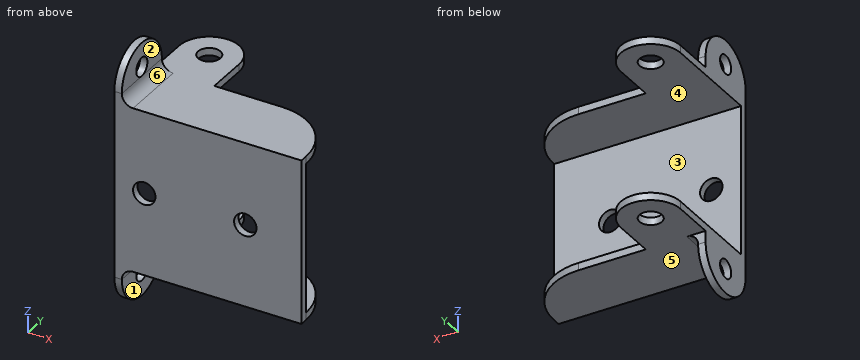
```python
from build123d import *

# Parameters (mm, degrees)
CROQUIS1_W              = 25
CROQUIS1_H              = 22
SALIENTE_EXTRUIR1_DEPTH = 1
CROQUIS2_W              = 8
CROQUIS2_H              = 1
SALIENTE_EXTRUIR2_DEPTH = 17.6
CROQUIS2_3_W            = 17
CROQUIS2_3_H            = 1
SALIENTE_EXTRUIR3_DEPTH = 8
REDONDEO2_RADIUS        = 4
REDONDEO2_LENGTH        = 1
REDONDEO3_R             = 8
REDONDEO4_RADIUS        = 4
REDONDEO4_LENGTH        = 1
CROQUIS4_R              = 1.5
CORTAR_EXTRUIR1_DEPTH   = 32.403980639
CROQUIS5_R              = 1.5
CORTAR_EXTRUIR2_DEPTH   = 25.22828925
CROQUIS6_W              = 1
CROQUIS6_H              = 9
SALIENTE_EXTRUIR4_DEPTH = 6
REDONDEO5_RADIUS        = 4.5
REDONDEO5_LENGTH        = 1
REDONDEO6_R             = 1.5
CORTAR_EXTRUIR3_REACH   = 37.496
CROQUIS7_R              = 1.25
CROQUIS8_W              = 25
CROQUIS8_H              = 11
CORTAR_EXTRUIR4_DEPTH   = 29.128455343


with BuildPart() as part:
    # Croquis1 → Saliente-Extruir1 (new body)
    with BuildSketch(Plane(origin=(0, 0, 0), x_dir=(1, 0, 0), z_dir=(0, 1, 0))):
        Rectangle(CROQUIS1_W, CROQUIS1_H)
    extrude(amount=SALIENTE_EXTRUIR1_DEPTH)

    # Croquis2 → Saliente-Extruir2 (add)
    with BuildSketch(Plane(origin=(0, 1, 0), x_dir=(1, 0, 0), z_dir=(0, 1, 0))):
        with Locations((-8.5, -10.5)):
            Rectangle(CROQUIS2_W, CROQUIS2_H)
        with Locations((-8.5, 10.5)):
            Rectangle(CROQUIS2_W, CROQUIS2_H)
    extrude(amount=SALIENTE_EXTRUIR2_DEPTH)

    # Croquis2<3> → Saliente-Extruir3 (add)
    with BuildSketch(Plane(origin=(0, 1, 0), x_dir=(1, 0, 0), z_dir=(0, 1, 0))):
        with Locations((4, 10.5)):
            Rectangle(CROQUIS2_3_W, CROQUIS2_3_H)
        with Locations((4, -10.5)):
            Rectangle(CROQUIS2_3_W, CROQUIS2_3_H)
    extrude(amount=SALIENTE_EXTRUIR3_DEPTH)

    # Redondeo2: full round fillet: the end face becomes a half cylinder, R = half its width
    redondeo2_face = Plane((-8.5, 18.6, 10.5), x_dir=(0, 0, -1), z_dir=(0, 1, 0))  # on the end face: x along it, z out of the body
    redondeo2_slab = redondeo2_face.offset(-REDONDEO2_RADIUS / 2) * Box(REDONDEO2_LENGTH, 2 * REDONDEO2_RADIUS, REDONDEO2_RADIUS, mode=Mode.PRIVATE)  # the body's end, R deep
    redondeo2_round = Plane((-8.5, 14.6, 10.5), x_dir=(0, 1, 0), z_dir=(0, 0, -1)) * Cylinder(REDONDEO2_RADIUS, REDONDEO2_LENGTH, mode=Mode.PRIVATE)  # its axis R under the face
    add(redondeo2_slab - redondeo2_round, mode=Mode.SUBTRACT)

    # Redondeo3
    redondeo3_edges = [part.edges().sort_by_distance(p)[0] for p in [
        (12.5, 9, 10.5),
        (12.5, 9, -10.5),
    ]]
    fillet(redondeo3_edges, radius=REDONDEO3_R)

    # Redondeo4: full round fillet: the end face becomes a half cylinder, R = half its width
    redondeo4_face = Plane((-8.5, 18.6, -10.5), x_dir=(0, 0, -1), z_dir=(0, 1, 0))  # on the end face: x along it, z out of the body
    redondeo4_slab = redondeo4_face.offset(-REDONDEO4_RADIUS / 2) * Box(REDONDEO4_LENGTH, 2 * REDONDEO4_RADIUS, REDONDEO4_RADIUS, mode=Mode.PRIVATE)  # the body's end, R deep
    redondeo4_round = Plane((-8.5, 14.6, -10.5), x_dir=(0, 1, 0), z_dir=(0, 0, -1)) * Cylinder(REDONDEO4_RADIUS, REDONDEO4_LENGTH, mode=Mode.PRIVATE)  # its axis R under the face
    add(redondeo4_slab - redondeo4_round, mode=Mode.SUBTRACT)

    # Croquis4 → Cortar-Extruir1 (cut, through all)
    with BuildSketch(Plane.XY.offset(11)):
        with Locations((-8.5, 14.6)):
            Circle(CROQUIS4_R)
    extrude(amount=-CORTAR_EXTRUIR1_DEPTH, mode=Mode.SUBTRACT)

    # Croquis5 → Cortar-Extruir2 (cut, through all)
    with BuildSketch(Plane(origin=(0, 1, 0), x_dir=(1, 0, 0), z_dir=(0, 1, 0))):
        with Locations(Location((5, 0, 0), (0, 0, 270))):
            Circle(CROQUIS5_R)
        with Locations(Location((-8.5, 0, 0), (0, 0, 270))):
            Circle(CROQUIS5_R)
    extrude(amount=-CORTAR_EXTRUIR2_DEPTH, mode=Mode.SUBTRACT)

    # Croquis6 → Saliente-Extruir4 (add)
    with BuildSketch(Plane.XY.offset(11)):
        with Locations((-12, 4.5)):
            Rectangle(CROQUIS6_W, CROQUIS6_H)
    extrude(amount=SALIENTE_EXTRUIR4_DEPTH)

    # Redondeo5: full round fillet: the end face becomes a half cylinder, R = half its width
    redondeo5_face = Plane((-12, 4.5, 17), x_dir=(1, 0, 0), z_dir=(0, 0, 1))  # on the end face: x along it, z out of the body
    redondeo5_slab = redondeo5_face.offset(-REDONDEO5_RADIUS / 2) * Box(REDONDEO5_LENGTH, 2 * REDONDEO5_RADIUS, REDONDEO5_RADIUS, mode=Mode.PRIVATE)  # the body's end, R deep
    redondeo5_round = Plane((-12, 4.5, 12.5), x_dir=(0, 0, 1), z_dir=(1, 0, 0)) * Cylinder(REDONDEO5_RADIUS, REDONDEO5_LENGTH, mode=Mode.PRIVATE)  # its axis R under the face
    add(redondeo5_slab - redondeo5_round, mode=Mode.SUBTRACT)

    # Redondeo6
    redondeo6_edges = [part.edges().sort_by_distance(p)[0] for p in [
        (-11.5, 4.5, 11),
    ]]
    fillet(redondeo6_edges, radius=REDONDEO6_R)

    # Croquis7 → Cortar-Extruir3 (cut, up to next)
    with BuildSketch(Plane.ZY.offset(12.5), mode=Mode.PRIVATE) as cortar_extruir3_sk1:
        with Locations((13.75, 4.5)):
            Circle(CROQUIS7_R)
    cortar_extruir3_tool1 = extrude(cortar_extruir3_sk1.sketch, amount=-CORTAR_EXTRUIR3_REACH, mode=Mode.PRIVATE) & part.part
    add(cortar_extruir3_tool1.solids().sort_by_distance((-12.5, 4.5, 13.75))[0], mode=Mode.SUBTRACT)

    # Croquis8 → Cortar-Extruir4 (cut, through all)
    with BuildSketch(Plane.XZ):
        with Locations((0, -5.5)):
            Rectangle(CROQUIS8_W, CROQUIS8_H)
    extrude(amount=-CORTAR_EXTRUIR4_DEPTH, mode=Mode.SUBTRACT)

    # Simetría1: part across plane


with BuildPart() as part_1:
    add(part.part)
    add(part.part.mirror(Plane.XY))


solid = part_1.part
```
Can you work these out from the model? Positions are in its coordinate system, mm. Face numbers are marked on the shaded views. A direction names the side the tool comes from. Round coordinates to 2 decimals unless told otherwise and drop trailing zeros. Loops run counter-clockwise (first coordinate to the right, second up) from the corner with the lowest first, then second, coordinate; pieces in that order, holes last. Notation, with made-up numbers: (23.25, 39) -> (60.25, 39) arc R9 ccw to (60.25, 45) -> close; hole circle Ø3 at (13, -13). An arc over 180 degrees is marked (long way). One line per item, written item: value. Start each with the question number.
1. For the marked faces 1, 2 and 3, which set-ups out of +Z, -Z, +X, -X, +Y, -Y let a thin tool reach every point of the face, with its end or its side?
2. If we mould it in two halves opening along Z, with no side actions, what happens to the marked faces 4, 5 and 6? For each: pulls with the +Z half, pulls with the -Z half, needs draft (parallel to the pull), parting line crosses it, or undercut.
3. For pin 1 (5.5 mm diameter, centred on x = 1.5, y = 6, fed in from -Z); pin 2 (1.8 mm diameter, centred on x = -8.5, z = 0, fed in from +Y); pin 3 (5 mm diameter, centred on x = 3.5, z = -6, fed in from +Y); pin 4 (1.5 mm diameter, centred on x = -5.5, z = -11, fed in from +Y), each with a flat end and sliding along its axis, tell me the tip position at first contact or that it passes through.
4. If we section it at A-A, the plane x = -8.5: Write out the boundary of the cut face in (y, z).
5. If we section it at B-B, the plane z = 0: Write out the boundary of the cut face in (x, y).
6. If we section it at D-D, the plane z = -13.75: Write out the boundary of the cut face in (x, y), then the cut area to 3 significant figures.
7. If we section it at C-C, the plane y = 11.5: Write out the boundary of the cut face in (x, z), then the cut area to 3 significant figures.
8. If I drill on probe 1 along Z at (x, y) = (-11.85, 4.5); probe 2 along Z at (x, y) = (5.5, 7.75); probe 3 along Y at (x, z) = (-8.5, -10.55), over which ranges is the centre line in solid material (lowest first)?
Calculated:
1. face 1: -Z, +X, +Y, -Y
1. face 2: +Z, +X, +Y, -Y
1. face 3: +X, -X, +Y
2. face 4: undercut
2. face 5: pulls with the -Z half
2. face 6: pulls with the +Z half
3. pin 1: stops at z = -11
3. pin 2: passes through
3. pin 3: stops at y = 1
3. pin 4: stops at y = 17.91
4. outline: (0, -11) -> (13.1, -11) -> (13.1, -10) -> (1, -10) -> (1, -1.5) -> (0, -1.5) -> close; (0, 1.5) -> (1, 1.5) -> (1, 10) -> (13.1, 10) -> (13.1, 11) -> (0, 11) -> close; (16.1, -11) -> (18.6, -11) -> (18.6, -10) -> (16.1, -10) -> close; (16.1, 10) -> (18.6, 10) -> (18.6, 11) -> (16.1, 11) -> close
5. outline: (-12.5, 0) -> (-10, 0) -> (-10, 1) -> (-12.5, 1) -> close; (-7, 0) -> (3.5, 0) -> (3.5, 1) -> (-7, 1) -> close; (6.5, 0) -> (12.5, 0) -> (12.5, 1) -> (6.5, 1) -> close
6. outline: (-12.5, 0.18) -> (-11.5, 0.18) -> (-11.5, 3.25) -> (-12.5, 3.25) -> close; (-12.5, 5.75) -> (-11.5, 5.75) -> (-11.5, 8.82) -> (-12.5, 8.82) -> close
6. area: 6.15 mm²
7. outline: (-12.5, -11) -> (-4.5, -11) -> (-4.5, -10) -> (-12.5, -10) -> close; (-12.5, 10) -> (-4.5, 10) -> (-4.5, 11) -> (-12.5, 11) -> close
7. area: 16.0 mm²
8. probe 1: z = -17 to -15, -12.5 to -10, 10 to 12.5, 15 to 17
8. probe 2: z = -11 to -10, 10 to 11
8. probe 3: y = 0 to 13.1, 16.1 to 18.6
